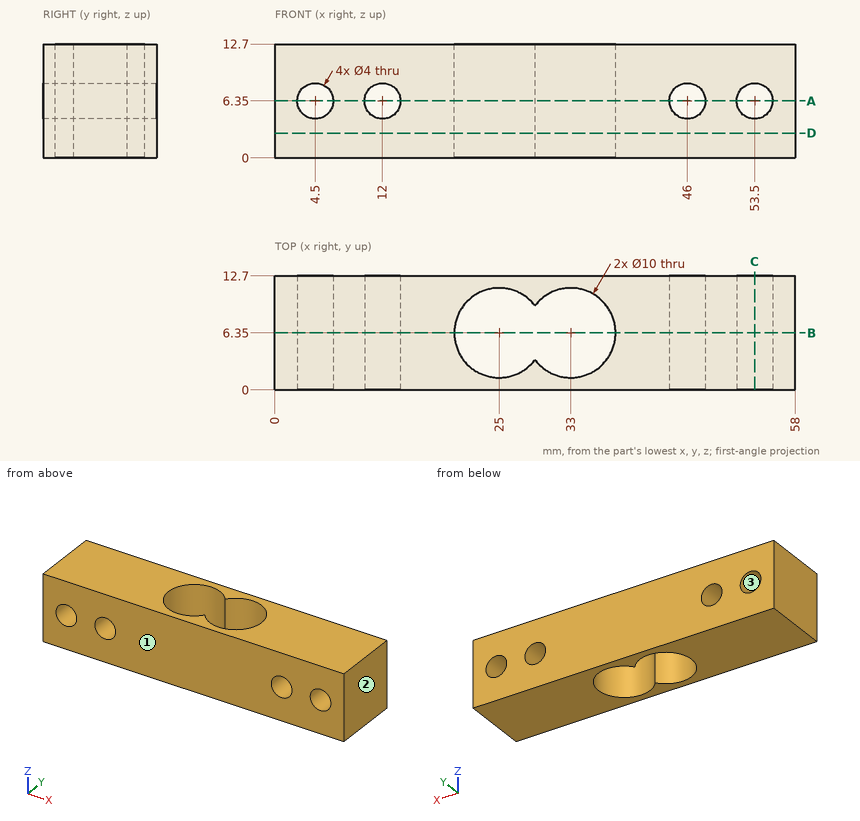
Study the drawing (mm; zero at the part's minimum x, y, z) and answer. Round coordinates to 2 decimals unless told otherwise and drop trailing zeros. Write each loop counter-clockwise with the first axis right and the second up, starting at its lowest first coordinate (ties: lowest second). Pieces come first, ordered by that corner, then holes.
1) A cutting plane is placed at D-D on z = 2.75. Determine the outline of the cut face in (x, y).
2) A cutting plane is placed at B-B on y = 6.35. Determine the outline of the cut face in (x, z).
3) Determine the mould class of the marked faces 1, 2 and 3 for opening direction X: pulls with the +X half, pulls with the -X half, needs draft (parallel to the pull), parting line crosses it, or undercut.
4) Consider probe 1 along X at (y, z) = (6.5, 4.25); probe 2 along Y at (x, z) = (33, 9.5); probe 3 along X at (y, z) = (6.35, 8). Determine where each line is inside the solid, lowest interval first.
5) A cutting plane is placed at C-C on x = 53.5. Determine the outline of the cut face in (y, z).
6) A cutting plane is placed at A-A on z = 6.35. Determine the outline of the cut face in (x, y).
Entries:
1. outline: (0, 0) - (58, 0) - (58, 12.7) - (0, 12.7) - close; hole (29, 3.35) arc R5 ccw (long way) to (29, 9.35) arc R5 ccw (long way) to start
2. outline: (0, 0) - (20, 0) - (20, 12.7) - (0, 12.7) - close; (38, 0) - (58, 0) - (58, 12.7) - (38, 12.7) - close; hole circle Ø4 at (4.5, 6.35); hole circle Ø4 at (12, 6.35); hole circle Ø4 at (46, 6.35); hole circle Ø4 at (53.5, 6.35)
3. face 1: needs draft
3. face 2: pulls with the +X half
3. face 3: undercut
4. probe 1: x = 0 to 20, 38 to 58
4. probe 2: y = 0 to 1.35, 11.35 to 12.7
4. probe 3: x = 0 to 3.37, 5.63 to 10.87, 13.13 to 20, 38 to 44.87, 47.13 to 52.37, 54.63 to 58
5. outline: (0, 0) - (12.7, 0) - (12.7, 4.35) - (0, 4.35) - close; (0, 8.35) - (12.7, 8.35) - (12.7, 12.7) - (0, 12.7) - close
6. outline: (0, 0) - (2.5, 0) - (2.5, 12.7) - (0, 12.7) - close; (6.5, 0) - (10, 0) - (10, 12.7) - (6.5, 12.7) - close; (14, 0) - (44, 0) - (44, 12.7) - (14, 12.7) - close; (48, 0) - (51.5, 0) - (51.5, 12.7) - (48, 12.7) - close; (55.5, 0) - (58, 0) - (58, 12.7) - (55.5, 12.7) - close; hole (29, 3.35) arc R5 ccw (long way) to (29, 9.35) arc R5 ccw (long way) to start
